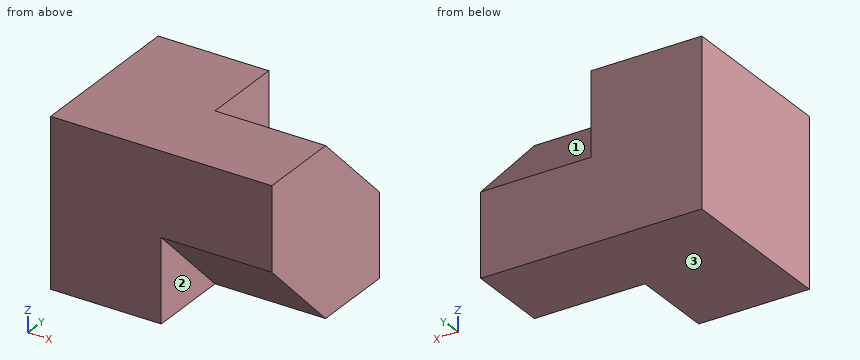
from build123d import *

# Parameters (mm, degrees)
F0_W     = 15
F0_H     = 15
F1_DEPTH = 20
F2_DEPTH = 40
F4_DEPTH = 20
F6_DEPTH = 20


with BuildPart() as f1:
    # F0 (on Right) → F1 (new body)
    with BuildSketch(Plane.YZ):
        with Locations((7.5, 7.5)):
            Rectangle(F0_W, F0_H)
        with Locations((22.5, 7.5)):
            Rectangle(F0_W, F0_H)
        with Locations((7.5, 22.5)):
            Rectangle(F0_W, F0_H)
        with Locations((22.5, 22.5)):
            Rectangle(F0_W, F0_H)
    extrude(amount=F1_DEPTH)

    # F0 (on Right) → F2 (join)
    with BuildSketch(Plane.YZ):
        with Locations((22.5, 7.5)):
            Rectangle(F0_W, F0_H)
        with Locations((22.5, 22.5)):
            Rectangle(F0_W, F0_H)
        with Locations((7.5, 22.5)):
            Rectangle(F0_W, F0_H)
    extrude(amount=F2_DEPTH)

    # F3 (on face) → F4 (cut)
    with BuildSketch(Plane.YZ.offset(40)):
        Polygon((30, 30), (15, 30), (30, 15), align=None)
    extrude(amount=-F4_DEPTH, mode=Mode.SUBTRACT)

    # F5 (on face) → F6 (join)
    with BuildSketch(Plane.YZ.offset(20)):
        Polygon((15, 15), (0, 15), (15, 0), align=None)
    extrude(amount=F6_DEPTH)


solid = f1.part
Input: part model. Units: mm. Frame: model coordinates. Face numbers are marked on the shaded views. A direction names the side the tool comes from. Coordinates: 2 decimals unless noted, no trailing zeros. Order: outer loops, then holes, each group sorted by start corner. A loop starts at its lowest first (then second) coordinate and runs counter-clockwise, first axis right, second up. Notation, with made-up numbers: M 2,-11 L 28,-11 A17 cw 28,-6 Z; hole C 63,-24.5 d5. An arc over 180 degrees is marked long. Write item = value, one per line. Start each with the question number.
(1) Section A-A on y = 7. Output: boundary loops of the cut face in (x, z), and give its area (3 significant figures).
(2) Line query: line 1 along X through (y, z) = (20.5, 28.75); line 2 along Z through (x, y) = (33, 21); line 3 along Z through (x, y) = (21, 16.25). Output: solid intervals per line, ascending. Write a range as [from, to].
(3) Section B-B on z = 11.75. Output: boundary loops of the cut face in (x, y), and give its area (4 significant figures).
(4) First-contact query: P1, Ø5, axis at x = 9.5, y = 3, coming from the -Z side; P2, Ø4.5, axis at y = 24, z = 24.5, coming from the +X side. Flat tips, straight axial feed; report the tip coordinate or a pass-through.
(5) Reachability of the marked faces 1, 2 and 3 from +Z, -Z, +X, -X, +Y, -Y: full face, straight path, thin tool, end or side. Return the list, or none.
Result set:
q1.outline = M 0,0 L 20,0 L 20,8 L 40,8 L 40,30 L 0,30 Z
q1.area = 1,040 mm²
q2.line_1 = [0, 20]
q2.line_2 = [0, 24]
q2.line_3 = [0, 28.75]
q3.outline = M 0,0 L 20,0 L 20,3.25 L 40,3.25 L 40,30 L 0,30 Z
q3.area = 1,135 mm²
q4.P1 = 0
q4.P2 = 20
q5.face_1 = +Z, +X, +Y
q5.face_2 = -Z, +X, -Y
q5.face_3 = -Z, +X, -X, +Y, -Y
